CAD build for the part. Positions are in the model's coordinates, mm. A direction names the side the tool comes from. Round coordinates to 2 decimals unless told otherwise and drop trailing zeros. Order: outer loops, then holes, each group sorted by start corner. A loop starts at its lowest first (then second) coordinate and runs counter-clockwise, first axis right, second up. Notation, with made-up numbers: M 28,87.5 L 79,87.5 A14 ccw 79,107.5 Z; hole C 82,-38.75 d4. An arc over 180 degrees is marked long. Answer as a JSON object with one key per item and string values. Group by question number.
```python
from build123d import *

# Parameters (mm, degrees)
PAD_DEPTH            = 17
POCKET_DEPTH         = 7
PAD001_DEPTH         = 3
PAD001_DEPTH_BACK    = 3
SKETCH003_R          = 1.1
POCKET001_DEPTH      = 5
POCKET001_DEPTH_BACK = -5
POCKET002_DEPTH      = 5
POCKET002_DEPTH_BACK = -5


with BuildPart() as part:
    # Sketch001 → Pad (new body)
    with BuildSketch(Plane.XY):
        with BuildLine():
            Line((-3, 3.354102), (-3, -3.354102))
            ThreePointArc((-3, -3.354102), (0, -4.5), (3, -3.354102))
            Line((3, 3.354102), (3, -3.354102))
            ThreePointArc((3, 3.354102), (0, 4.5), (-3, 3.354102))
        make_face()
    extrude(amount=PAD_DEPTH)

    # Sketch → Pocket (cut)
    with BuildSketch(Plane.XY):
        with BuildLine():
            Line((1.5, 2), (1.5, -2))
            ThreePointArc((-1.5, -2), (0, -2.5), (1.5, -2))
            Line((-1.5, 2), (-1.5, -2))
            ThreePointArc((1.5, 2), (0, 2.5), (-1.5, 2))
        make_face()
    extrude(amount=POCKET_DEPTH, mode=Mode.SUBTRACT)

    # Sketch002 → Pad001 (join, two sides)
    with BuildSketch(Plane.YZ) as pad001_sk:
        with BuildLine():
            Line((-10.5, 17), (10.5, 17))
            ThreePointArc((10.5, 17), (11.914214, 17.585786), (12.5, 19))
            Line((12.5, 55), (12.5, 19))
            ThreePointArc((12.5, 55), (11.914214, 56.414214), (10.5, 57))
            Line((-10.5, 57), (10.5, 57))
            ThreePointArc((-10.5, 57), (-11.914214, 56.414214), (-12.5, 55))
            Line((-12.5, 55), (-12.5, 19))
            ThreePointArc((-12.5, 19), (-11.914214, 17.585786), (-10.5, 17))
        make_face()
    extrude(amount=PAD001_DEPTH)
    extrude(pad001_sk.sketch, amount=-PAD001_DEPTH_BACK)

    # Sketch003 → Pocket001 (cut, two sides)
    with BuildSketch(Plane.YZ) as pocket001_sk:
        with Locations((-10.5, 55)):
            Circle(SKETCH003_R)
        with Locations((10.5, 55)):
            Circle(SKETCH003_R)
        with Locations((10.5, 41.5)):
            Circle(SKETCH003_R)
        with Locations((-10.5, 41.5)):
            Circle(SKETCH003_R)
    extrude(amount=-POCKET001_DEPTH, mode=Mode.SUBTRACT)
    extrude(pocket001_sk.sketch, amount=-POCKET001_DEPTH_BACK, mode=Mode.SUBTRACT)

    # Sketch004 → Pocket002 (cut, two sides)
    with BuildSketch(Plane.YZ) as pocket002_sk:
        with BuildLine():
            Line((-9.4, 28.5), (9.4, 28.5))
            ThreePointArc((10.4, 27.5), (10.107107, 28.207107), (9.4, 28.5))
            Line((10.4, 27.5), (10.4, 22.5))
            ThreePointArc((9.4, 21.5), (10.107107, 21.792893), (10.4, 22.5))
            Line((9.4, 21.5), (-9.4, 21.5))
            ThreePointArc((-10.4, 22.5), (-10.107107, 21.792893), (-9.4, 21.5))
            Line((-10.4, 27.5), (-10.4, 22.5))
            ThreePointArc((-9.4, 28.5), (-10.107107, 28.207107), (-10.4, 27.5))
        make_face()
    extrude(amount=-POCKET002_DEPTH, mode=Mode.SUBTRACT)
    extrude(pocket002_sk.sketch, amount=-POCKET002_DEPTH_BACK, mode=Mode.SUBTRACT)


solid = part.part
```
Item 1: Cut at B-B, the plane z = 41.5. Give the cut face in (x, y).
Item 2: Cut at A-A, the plane y = -7.5. Give the cut face in (x, z), and give its area (3 significant figures).
Item 3: 3-axis set-ups, long thin cutter, end or side, ignore diameter. For faces 1 (the face through (0, 0, 21.5)), 2 (the face through (0, -4.5, 8.4)), 3 (the face through (-1.5, 0, 3)): which of +Z, -Z, +X, -X, +Y, -Y reach the whole face in a straight line?
Item 4: Cut at C-C, the plane x = -0.25. Give the cut face in (y, z).
Item 5: Cut at D-D, the plane z = 15. Give the cut face in (x, y), and give its area (3 significant figures).
Item 6: Two-plate mould, pull along Y, no slides. Class faces 4 (the face through (0, -12.5, 37)), 5 (the face through (-0.042, -10.099, 28.215)), 6 (the face through (0.04, 10.36, 56.09)), 7 (the face through (0, 12.5, 37)): +Y half, -Y half, draft (parallel to the pull), parting line (faces both ways), or undercut.
Item 7: Drill centre lines: line 1 (Z direction, x = 1.05, y = -10.5); line 2 (Y direction, x = -0.4, z = 41.5); line 3 (Z direction, x = 0.25, y = 0). Where is each one in solid material? Low to high. Write a range as [from, to].
Item 8: Flat gauge pins, fed straight in: pin 1 Ø1.3 at (y, z) = (10.5, 55) entering from +X; pin 2 Ø1 at (x, z) = (-2, 12) entering from +Y; pin 3 Ø1.5 at (x, y) = (0, -8.5) entering from -Z; pin 4 Ø0.9 at (x, y) = (0.5, -0.5) entering from -Z. Where does each tip first touch, or does it go through?
Response values:
{
 "1": {"outline": "M -3,-12.5 L 3,-12.5 L 3,-11.6 L -3,-11.6 Z; M -3,-9.4 L 3,-9.4 L 3,9.4 L -3,9.4 Z; M -3,11.6 L 3,11.6 L 3,12.5 L -3,12.5 Z"},
 "2": {"outline": "M -3,17 L 3,17 L 3,21.5 L -3,21.5 Z; M -3,28.5 L 3,28.5 L 3,57 L -3,57 Z", "area": "198 mm^2"},
 "3": {"face 1": "+X, -X", "face 2": "-Z, -Y", "face 3": "-Z"},
 "4": {"outline": "M -12.5,19 A2 ccw -10.5,17 L -4.49,17 L -4.49,0 L -2.49,0 L -2.49,7 L 2.49,7 L 2.49,0 L 4.49,0 L 4.49,17 L 10.5,17 A2 ccw 12.5,19 L 12.5,55 A2 ccw 10.5,57 L -10.5,57 A2 ccw -12.5,55 Z; hole C -10.5,41.5 d2.2; hole C -10.5,55 d2.2; hole M -10.4,22.5 A1 ccw -9.4,21.5 L 9.4,21.5 A1 ccw 10.4,22.5 L 10.4,27.5 A1 ccw 9.4,28.5 L -9.4,28.5 A1 ccw -10.4,27.5 Z; hole C 10.5,41.5 d2.2; hole C 10.5,55 d2.2"},
 "5": {"outline": "M -3,-3.35 A4.5 ccw 3,-3.35 L 3,3.35 A4.5 ccw -3,3.35 Z", "area": "49.7 mm^2"},
 "6": {"face 4": "-Y half", "face 5": "undercut", "face 6": "undercut", "face 7": "+Y half"},
 "7": {"line 1": "[17, 40.4], [42.6, 53.9], [56.1, 57]", "line 2": "[-12.5, -11.6], [-9.4, 9.4], [11.6, 12.5]", "line 3": "[7, 21.5], [28.5, 57]"},
 "8": {"pin 1": "through", "pin 2": "y = 4.24", "pin 3": "z = 17", "pin 4": "z = 7"}
}
